```python
from build123d import *

# Parameters (mm, degrees)
SALIENTE_EXTRUIR1_DEPTH = 3
CROQUIS3_R              = 2
CROQUIS3_W              = 40
CROQUIS3_H              = 20
CORTAR_EXTRUIR1_DEPTH   = 4
REDONDEO1_R             = 1
CROQUIS4_R              = 1.5
CORTAR_EXTRUIR2_DEPTH   = 3


with BuildPart() as part:
    # Croquis1 → Saliente-Extruir1 (new body)
    with BuildSketch(Plane.XY):
        Polygon((75, 13.5), (15, 13.5), (15, 10), (-15, 10), (-15, 13.5), (-75, 13.5), (-75, -13.5), (-15, -13.5), (-15, -10), (15, -10), (15, -13.5), (75, -13.5), align=None)
    extrude(amount=SALIENTE_EXTRUIR1_DEPTH)

    # Croquis3 → Cortar-Extruir1 (cut, through all)
    with BuildSketch(Plane.XY.offset(3)):
        with Locations((-21.75, -5)):
            Circle(CROQUIS3_R)
        with Locations((-21.75, 5)):
            Circle(CROQUIS3_R)
        with Locations((-72.25, -5)):
            Circle(CROQUIS3_R)
        with Locations((-72.25, 5)):
            Circle(CROQUIS3_R)
        with Locations((72.25, 5)):
            Circle(CROQUIS3_R)
        with Locations((72.25, -5)):
            Circle(CROQUIS3_R)
        with Locations((21.75, 5)):
            Circle(CROQUIS3_R)
        with Locations((21.75, -5)):
            Circle(CROQUIS3_R)
        with Locations((-47, 0)):
            Rectangle(CROQUIS3_W, CROQUIS3_H)
        with Locations((47, 0)):
            Rectangle(CROQUIS3_W, CROQUIS3_H)
    extrude(amount=-CORTAR_EXTRUIR1_DEPTH, mode=Mode.SUBTRACT)

    # Redondeo1
    redondeo1_edges = [part.edges().sort_by_distance(p)[0] for p in [
        (-75, -13.5, 1.5),
        (-75, 13.5, 1.5),
        (-15, 13.5, 1.5),
        (-15, 10, 1.5),
        (15, 10, 1.5),
        (15, 13.5, 1.5),
        (75, 13.5, 1.5),
        (75, -13.5, 1.5),
        (15, -13.5, 1.5),
        (15, -10, 1.5),
        (-15, -10, 1.5),
        (-15, -13.5, 1.5),
    ]]
    fillet(redondeo1_edges, radius=REDONDEO1_R)

    # Croquis4 → Cortar-Extruir2 (cut)
    with BuildSketch(Plane.XY.offset(3)):
        with Locations((15, 0)):
            Circle(CROQUIS4_R)
        with Locations((-15, 0)):
            Circle(CROQUIS4_R)
    extrude(amount=-CORTAR_EXTRUIR2_DEPTH, mode=Mode.SUBTRACT)


solid = part.part
```
Could you check a few things on this model? Use its own coordinates, in mm. A direction names the side the tool comes from. Coordinates: 2 decimals unless noted, no trailing zeros. Loops run counter-clockwise (first coordinate to the right, second up) from the corner with the lowest first, then second, coordinate; pieces in that order, holes last.
1) Imagine slicing it at A-A (y = 0). List the corners of the cut face in (x, z) for me, and give its area (3 significant figures).
Reported:
outline: (-75, 0) - (-67, 0) - (-67, 3) - (-75, 3) - close; (-27, 0) - (-16.5, 0) - (-16.5, 3) - (-27, 3) - close; (-13.5, 0) - (13.5, 0) - (13.5, 3) - (-13.5, 3) - close; (16.5, 0) - (27, 0) - (27, 3) - (16.5, 3) - close; (67, 0) - (75, 0) - (75, 3) - (67, 3) - close
area: 192 mm2
2) Thinking about a two-plate mould opening in X: for faces 1 (the face through (-16.5, 0.07, 1.52)), 2 (the face through (45, -13.5, 1)), 3 (the face through (75, 0, 1)), which applies, released by +X, released by -X, zero draft, split by the parting line, or undercut?
Reported:
face 1: undercut
face 2: zero draft
face 3: released by +X
3) Imagine slicing it at C-C (z = 2). State how many separate pieces and enclosed holes the cut face has, and give its area (3 significant figures).
Reported:
separate pieces: 1
enclosed holes: 12
area: 2,120 mm2
4) Please list where these lines run through material, in increasing order: line 1 along X through (y, z) = (-2.75, 0.75); line 2 along Y through (x, z) = (21.75, 1); line 3 along X through (y, z) = (-11, 0.6).
Reported:
line 1: x = -75 to -67, -27 to 27, 67 to 75
line 2: y = -13.5 to -7, -3 to 3, 7 to 13.5
line 3: x = -75 to -15, 15 to 75
5) Which directions (+Z, -Z, +X, -X, +Y, -Y) give clear straight access to the entire face, cutting with the end or side of a thin tool? Please do faces 4 (the face through (45, 13.5, 1)), 5 (the face through (0, -10, 1)), 6 (the face through (-18, 0, 3)), 7 (the face through (47, -10, 2)), 8 (the face through (0, 10, 1)).
Reported:
face 4: +Z, -Z, +X, -X, +Y
face 5: +Z, -Z, -Y
face 6: +Z, +X, -X, +Y, -Y
face 7: +Z, -Z
face 8: +Z, -Z, +Y
6) Imagine slicing it at B-B (x = -31.5). List the corners of the cut face in (y, z) for me, and give its area (3 significant figures).
Reported:
outline: (-13.5, 0) - (-10, 0) - (-10, 3) - (-13.5, 3) - close; (10, 0) - (13.5, 0) - (13.5, 3) - (10, 3) - close
area: 21.0 mm2
7) Imagine slicing it at D-D (x = 10.5). List the corners of the cut face in (y, z) for me, and give its area (3 significant figures).
Reported:
outline: (-10, 0) - (10, 0) - (10, 3) - (-10, 3) - close
area: 60.0 mm2
8) Will this pin go through, and if not, where does the flat tip stop? pin 1 Ø1.5 at (x, z) = (-0.5, 2.5) entering from -Y.
Reported:
pin 1: stops at y = -10
